Can you work these out from the model? Positions are in its coordinate system, mm. Face numbers are marked on the shaded views. A direction names the side the tool comes from. Coordinates: 2 decimals unless noted, no trailing zeros. Write each loop counter-clockwise with the first axis right and the second up, starting at its lowest first coordinate (ties: lowest second). Pieces come first, ordered by that corner, then holes. Notation, with made-up numbers: (22.5, -26) - (47.5, -26) arc R14 ccw to (47.5, -17) - close; hole circle Ø5 at (31.25, 78). An arc over 180 degrees is marked (long way). Use one line per item in the form item = value. Start each with the question number.
(1) For pin 1 Ø1.2 at (x, y) = (0, 0) entering from -Z; pin 2 Ø1.5 at (y, z) = (-1, 11) entering from +X; pin 3 Ø2 at (x, z) = (1.5, -3) entering from +Y, each with a flat end and sliding along its axis, tell me the tip position at first contact or that it passes through.
(2) If we section it at A-A on x = 0: Please give me the cut outline in (y, z).
(3) If I drill on probe 1 along Y at (x, z) = (0, -6); probe 2 along Z at (x, y) = (2.2, -0.2); probe 3 along Y at (x, z) = (0, -3), over which ranges is the centre line in solid material (lowest first)? Write a range as from..to.
(4) If we section it at C-C on z = -2: Please give me the cut outline in (x, y), then the cut area to 3 significant figures.
(5) On a 3-axis mill with a long thin cutter (end or side, diameter ignored), from which of +Z, -Z, +X, -X, +Y, -Y can I reach the whole of each face in a straight line? I mean the marked faces 1 and 2. Say none if no direction works.
(6) If we section it at D-D on z = 16: Please give me the cut outline in (x, y), then the cut area to 3 significant figures.
```python
from build123d import *

# Parameters (mm, degrees)
F0_R     = 2.5
F1_DEPTH = 25
F2_R     = 1.5
F3_DEPTH = 5
F4_R     = 2.5
F4_R_2   = 1.5
F5_DEPTH = 10
F7_D     = 2
F8_SIZE  = 0.2


with BuildPart() as f1:
    # F0 (on Top) → F1 (new body)
    with BuildSketch(Plane.XY):
        Circle(F0_R)
    extrude(amount=F1_DEPTH)

    # F2 (on face) → F3 (join)
    with BuildSketch(Plane(origin=(0, 0, 0), x_dir=(1, 0, 0), z_dir=(0, 0, -1))):
        Circle(F2_R)
    extrude(amount=F3_DEPTH)

    # F4 (on face) → F5 (join)
    with BuildSketch(Plane(origin=(0, 0, -5), x_dir=(1, 0, 0), z_dir=(0, 0, -1))):
        Circle(F4_R)
        Circle(F4_R_2, mode=Mode.SUBTRACT)
        Circle(F4_R_2)
    extrude(amount=F5_DEPTH)

    # F7 (through all)
    with Locations(Plane.XY.offset(25)):
        with Locations((0, 0)):
            Hole(F7_D / 2)

    # F8
    f8_edges = [f1.edges().sort_by_distance(p)[0] for p in [
        (-2.5, 0, 25),
        (-2.5, 0, -5),
        (-2.5, 0, -15),
        (-2.5, 0, 0),
    ]]
    chamfer(f8_edges, length=F8_SIZE)


solid = f1.part
```
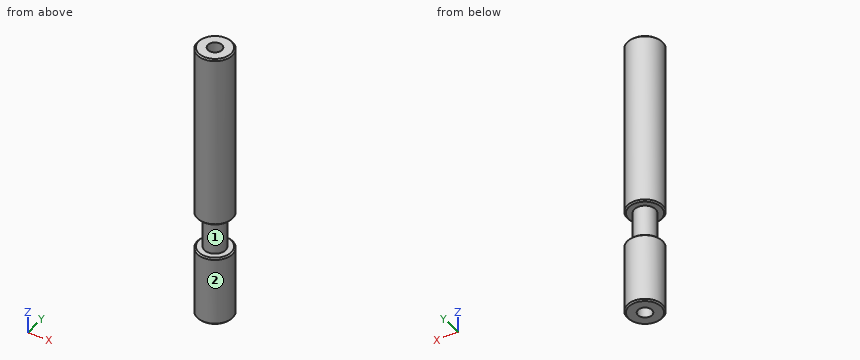
Reported:
q1.pin_1 = through
q1.pin_2 = 2.49
q1.pin_3 = 1.41
q2.outline = (-2.5, -14.8) - (-2.3, -15) - (-1, -15) - (-1, 25) - (-2.3, 25) - (-2.5, 24.8) - (-2.5, 0.2) - (-2.3, 0) - (-1.5, 0) - (-1.5, -5) - (-2.3, -5) - (-2.5, -5.2) - close; (1, -15) - (2.3, -15) - (2.5, -14.8) - (2.5, -5.2) - (2.3, -5) - (1.5, -5) - (1.5, 0) - (2.3, 0) - (2.5, 0.2) - (2.5, 24.8) - (2.3, 25) - (1, 25) - close
q3.probe_1 = -2.5..-1, 1..2.5
q3.probe_2 = -15..-5, 0..25
q3.probe_3 = -1.5..-1, 1..1.5
q4.outline = circle Ø3 at (0, 0); hole circle Ø2 at (0, 0)
q4.area = 3.93 mm2
q5.face_1 = none
q5.face_2 = +Z, -Z
q6.outline = circle Ø5 at (0, 0); hole circle Ø2 at (0, 0)
q6.area = 16.5 mm2
